```python
from build123d import *

# Parameters (mm, degrees)
SKETCH2_R           = 12.5
SKETCH2_R_2         = 4
BOSS_EXTRUDE1_DEPTH = 3.5
SKETCH3_R           = 5
SKETCH3_R_2         = 4
BOSS_EXTRUDE2_DEPTH = 2
SKETCH4_R           = 5
SKETCH4_R_2         = 4
BOSS_EXTRUDE3_DEPTH = 5
SKETCH5_R           = 1.6
CUT_EXTRUDE1_DEPTH  = 9.5


with BuildPart() as part:
    # Sketch2 → Boss-Extrude1 (new body)
    with BuildSketch(Plane(origin=(0, 0, 0), x_dir=(1, 0, 0), z_dir=(0, 1, 0))):
        Circle(SKETCH2_R)
        Circle(SKETCH2_R_2, mode=Mode.SUBTRACT)
    extrude(amount=BOSS_EXTRUDE1_DEPTH)

    # Sketch3 → Boss-Extrude2 (add)
    with BuildSketch(Plane(origin=(0, 3.5, 0), x_dir=(1, 0, 0), z_dir=(0, 1, 0))):
        Circle(SKETCH3_R)
        Circle(SKETCH3_R_2, mode=Mode.SUBTRACT)
    extrude(amount=BOSS_EXTRUDE2_DEPTH)

    # Sketch4 → Boss-Extrude3 (add)
    with BuildSketch(Plane.XZ):
        Circle(SKETCH4_R)
        Circle(SKETCH4_R_2, mode=Mode.SUBTRACT)
    extrude(amount=BOSS_EXTRUDE3_DEPTH)

    # Sketch5 → Cut-Extrude1 (cut, through all)
    with BuildSketch(Plane(origin=(0, 3.5, 0), x_dir=(1, 0, 0), z_dir=(0, 1, 0))):
        with Locations((0, 8)):
            Circle(SKETCH5_R)
        with Locations((8, 0)):
            Circle(SKETCH5_R)
        with Locations((0, -8)):
            Circle(SKETCH5_R)
        with Locations((-8, 0)):
            Circle(SKETCH5_R)
    extrude(amount=-CUT_EXTRUDE1_DEPTH, mode=Mode.SUBTRACT)


solid = part.part
```
Check sheet for the modelled part. Datum: model origin and axes. Units: mm. A direction names the side the tool comes from. Give positions to 0.01 mm unless a question says otherwise; leave off trailing zeros. Write each loop counter-clockwise with the first axis right and the second up, starting at its lowest first coordinate (ties: lowest second). Pieces come first, ordered by that corner, then holes. Notation, with made-up numbers: (22, 43.25) - (48, 43.25) arc R9 cw to (48, 48.25) - close; hole circle Ø1 at (19, -6.5). An arc over 180 degrees is marked (long way). Answer as a JSON object with one key per item and string values. Group by question number.
1) Sectioned sample at A-A (z = 0). Record the cut outline in (x, y), then the cut area to 3 significant figures.
2) Thickness scan on probe 1 along Z at (x, y) = (0, 2.35); probe 2 along Z at (x, y) = (-8, 1.4). Record the ranges inside material, lowest first. Write a range as from..to.
3) Sectioned sample at C-C (x = 8). Record the cut outline in (y, z).
4) Depth check by flat-ended pin: P1, Ø1.5, axis at x = -5.5, y = 4, coming from the +Z side; P2, Ø10, axis at x = 7, z = -8, coming from the -Y side; P3, Ø3.5, axis at x = -8, z = 0, coming from the +Y side; P4, Ø1.9, axis at x = 0, z = -8, coming from the +Y side. Enter the tip coordinate at first touch or a pass-through.
5) Sectioned sample at B-B (x = 0). Record the cut outline in (y, z), then the cut area to 3 significant figures.
6) Access from +Z, -Z, +X, -X, +Y, -Y to the whole of each face (thin tool, end or side, straight path). Record for faces 4 (the face through (-9.6, 1.77, -0.07)), 5 (the face through (-1.08, -2.46, -4.88)), 6 (the face through (-1.08, 4.49, 4.88)).
7) Release check for a two-part mould opening along X. For faces 1 (the face through (-0.2, 0, 5.4)), 2 (the face through (11.923, 1.726, -3.755)), 3 (the face through (-0.35, 1.77, 9.56)) record: pulls with the +X half, pulls with the -X half, needs draft (parallel to the pull), parting line crosses it, or undercut.
8) Sectioned sample at D-D (z = -8). Record the cut outline in (x, y), then the cut area to 3 significant figures.
Geometry results:
{
 "1": {"outline": "(-12.5, 0) - (-9.6, 0) - (-9.6, 3.5) - (-12.5, 3.5) - close; (-6.4, 0) - (-5, 0) - (-5, -5) - (-4, -5) - (-4, 5.5) - (-5, 5.5) - (-5, 3.5) - (-6.4, 3.5) - close; (4, -5) - (5, -5) - (5, 0) - (6.4, 0) - (6.4, 3.5) - (5, 3.5) - (5, 5.5) - (4, 5.5) - close; (9.6, 0) - (12.5, 0) - (12.5, 3.5) - (9.6, 3.5) - close", "area": "51.1 mm^2"},
 "2": {"probe 1": "z = -12.5..-9.6, -6.4..-4, 4..6.4, 9.6..12.5", "probe 2": "z = -9.6..-1.6, 1.6..9.6"},
 "3": {"outline": "(0, -9.6) - (3.5, -9.6) - (3.5, -1.6) - (0, -1.6) - close; (0, 1.6) - (3.5, 1.6) - (3.5, 9.6) - (0, 9.6) - close"},
 "4": {"P1": "stops at z = 11.48", "P2": "stops at y = 0", "P3": "stops at y = 3.5", "P4": "passes through"},
 "5": {"outline": "(-5, -5) - (0, -5) - (0, -6.4) - (3.5, -6.4) - (3.5, -5) - (5.5, -5) - (5.5, -4) - (-5, -4) - close; (-5, 4) - (5.5, 4) - (5.5, 5) - (3.5, 5) - (3.5, 6.4) - (0, 6.4) - (0, 5) - (-5, 5) - close; (0, -12.5) - (3.5, -12.5) - (3.5, -9.6) - (0, -9.6) - close; (0, 9.6) - (3.5, 9.6) - (3.5, 12.5) - (0, 12.5) - close", "area": "51.1 mm^2"},
 "6": {"face 4": "+Y, -Y", "face 5": "-Y", "face 6": "+Y"},
 "7": {"face 1": "needs draft", "face 2": "parting line crosses it", "face 3": "undercut"},
 "8": {"outline": "(-9.6, 0) - (-1.6, 0) - (-1.6, 3.5) - (-9.6, 3.5) - close; (1.6, 0) - (9.6, 0) - (9.6, 3.5) - (1.6, 3.5) - close", "area": "56.0 mm^2"}
}
